```python
from build123d import *

# Parameters (mm, degrees)
F1_DEPTH      = 3.5
F2_R          = 1.25
F3_DEPTH      = 25
F3_DEPTH_BACK = 25
F4_T4_DEPTH   = 12.7513736877
F4_T9_DEPTH   = 12.4486649129


# Not quite as in the source:
# - a fillet or chamfer that OpenCascade refuses, or shapes differently, is made with other operations: its cross-section is extruded or revolved along the edge and cut away or added


with BuildPart() as f1:
    # F0 (on Top) → F1 (new body)
    with BuildSketch(Plane.XY):
        Polygon((-9.9924615563, -3.7976490931), (11.3075384437, -3.7976490931), (11.3075384437, 4.1987212708), (11.6869780256, 4.1973420195), (11.6869780256, 5.1973420195), (-10.3793237358, 5.1973420195), (-10.3752534696, 4.2007874551), (-9.9924615563, 4.2023509069), align=None)
        Polygon((11.6869780256, 5.1973420195), (11.6869780256, 4.1973420195), (14.0588939546, 4.1887201777), (14.0588939546, 9.6923498138), (-12.4411060454, 9.6923498138), (-12.4411060454, 4.1923498138), (-10.3752534696, 4.2007874551), (-10.3793237358, 5.1973420195), (-11.1709162593, 5.1973420195), (-11.1709162593, 8.1973420195), (12.6290837407, 8.1973420195), (12.6290837407, 5.1973420195), align=None)
    extrude(amount=F1_DEPTH)

    # F2 (on Right) → F3 (cut, two sides)
    with BuildSketch(Plane.YZ) as f3_sk:
        with Locations((-2.1757856011, 1.7836129991)):
            Circle(F2_R)
    extrude(amount=-F3_DEPTH, mode=Mode.SUBTRACT)
    extrude(f3_sk.sketch, amount=F3_DEPTH_BACK, mode=Mode.SUBTRACT)

    # F4: fillet of radius 2 on 2 edges, made by hand


with BuildPart() as f4_tool2:
    # F4_s3 → F4_t4 (new body)
    with BuildSketch(Plane(origin=(6.2921600495, -0.0228718094, 0), x_dir=(0, 0, 1), z_dir=(0.9999933936, -0.0036349454, 0))):
        with BuildLine():
            ThreePointArc((3.5, -6.2397958172), (2.9142135624, -4.8255822548), (1.5, -4.2397958172))
            Line((1.5, -4.2397958172), (3.5, -4.2397958172))
            Line((3.5, -4.2397958172), (3.5, -6.2397958172))
        make_face()
    extrude(amount=F4_T4_DEPTH)

    split(bisect_by=Plane.YZ.offset(11.3075384437), keep=Keep.TOP)


with BuildPart() as f1_1:
    add(f1.part)

    # F4_t1: cut F4_tool2
    add(f4_tool2.part, mode=Mode.SUBTRACT)


with BuildPart() as f4_tool7:
    # F4_s8 → F4_t9 (new body)
    with BuildSketch(Plane(origin=(-17.423734114, -0.0711644294, 0), x_dir=(0, 0, 1), z_dir=(0.9999916592, 0.0040843045, 0))):
        with BuildLine():
            ThreePointArc((3.5, -6.2431281117), (2.9142135624, -4.8289145493), (1.5, -4.2431281117))
            Line((1.5, -4.2431281117), (3.5, -4.2431281117))
            Line((3.5, -4.2431281117), (3.5, -6.2431281117))
        make_face()
    extrude(amount=F4_T9_DEPTH)

    split(bisect_by=Plane.YZ.offset(-9.9924615563), keep=Keep.BOTTOM)


with BuildPart() as f1_2:
    add(f1_1.part)

    # F4_t6: cut F4_tool7
    add(f4_tool7.part, mode=Mode.SUBTRACT)


solid = f1_2.part
```
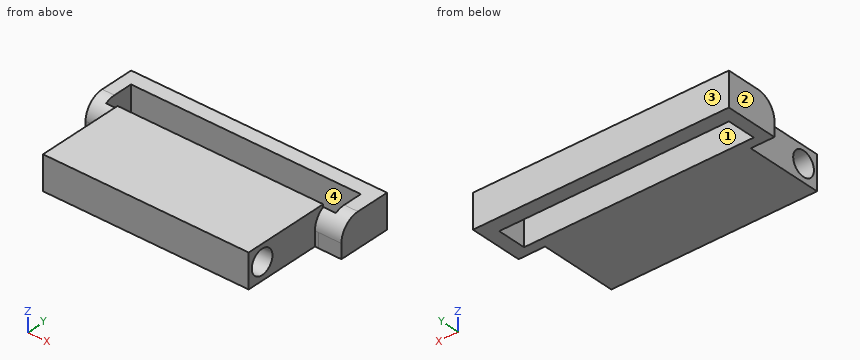
Model file for the job. Use its own axes, mm. Face numbers are marked on the shaded views. A direction names the side the tool comes from. Round coordinates to 2 decimals unless told otherwise and drop trailing zeros. Write each loop counter-clockwise with the first axis right and the second up, starting at its lowest first coordinate (ties: lowest second). Pieces come first, ordered by that corner, then holes. Notation, with made-up numbers: (17.25, -8.75) -> (52.25, -8.75) arc R23 cw to (52.25, 14.25) -> close; hole circle Ø3 at (74.25, -1.75). An arc over 180 degrees is marked (long way). Answer as CSV lines item,"result".
1. Tool access for the marked faces 3 and 4: list every direction of +Z, -Z, +X, -X, +Y, -Y with a clear straight run to the whole face (end or side of a thin tool).
Resolved:
face 3,"+Z, -Z, +X, -X, +Y"
face 4,"+Z, -Z"
2. Pin check, flat tips, straight feed: pin 1 Ø2 at (y, z) = (-2.18, 1.78) entering from -X; pin 2 Ø1.8 at (y, z) = (2, 1.5) entering from +X. Stop position of each tip, or through.
Resolved:
pin 1,"through"
pin 2,"x = 11.31"
3. Slice it at D-D, the plane y = -1.5. List the corners of the cut face in (x, z).
Resolved:
outline,"(-9.99, 0) -> (11.31, 0) -> (11.31, 0.73) -> (-9.99, 0.73) -> close; (-9.99, 2.84) -> (11.31, 2.84) -> (11.31, 3.5) -> (-9.99, 3.5) -> close"
4. Drill centre lines: line 1 (Y direction, x = 5, z = 1.75); line 2 (Y direction, x = -4.5, z = 2.6); line 3 (X direction, y = 6, z = 1). Where is each one in solid material? Low to high.
Resolved:
line 1,"-3.8 to -3.43, -0.93 to 5.2, 8.2 to 9.69"
line 2,"-3.8 to -3.12, -1.23 to 5.2, 8.2 to 9.69"
line 3,"-12.44 to -11.17, 12.63 to 14.06"
5. Slice it at A-A, the plane y = 6.5. List the corners of the cut face in (x, z), plus the area to 3 significant figures.
Resolved:
outline,"(-12.44, 0) -> (-11.17, 0) -> (-11.17, 3.5) -> (-12.44, 3.5) -> close; (12.63, 0) -> (14.06, 0) -> (14.06, 3.5) -> (12.63, 3.5) -> close"
area,"9.45 mm²"
6. Slice it at C-C, the plane x = -1.5. List the corners of the cut face in (y, z), plus the area to 3 significant figures.
Resolved:
outline,"(-3.8, 0) -> (5.2, 0) -> (5.2, 3.5) -> (-3.8, 3.5) -> close; (8.2, 0) -> (9.69, 0) -> (9.69, 3.5) -> (8.2, 3.5) -> close; hole circle Ø2.5 at (-2.18, 1.78)"
area,"31.8 mm²"
7. Slice it at B-B, the plane z = 1.2. List the corners of the cut face in (x, y), plus the area to 3 significant figures.
Resolved:
outline,"(-12.44, 4.19) -> (-9.99, 4.2) -> (-9.99, -1.07) -> (11.31, -1.07) -> (11.31, 4.2) -> (14.06, 4.19) -> (14.06, 9.69) -> (-12.44, 9.69) -> close; (-9.99, -3.8) -> (11.31, -3.8) -> (11.31, -3.28) -> (-9.99, -3.28) -> close; hole (-11.17, 5.2) -> (12.63, 5.2) -> (12.63, 8.2) -> (-11.17, 8.2) -> close"
area,"197 mm²"
8. Mould opens along X. For the marked faces 1 and 2 say: +X half, -X half, draft (parallel to the pull), parting line (faces both ways), or undercut.
Resolved:
face 1,"undercut"
face 2,"-X half"
